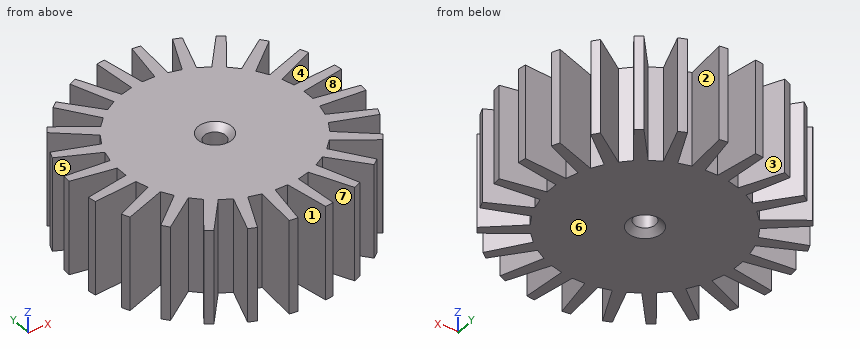
from build123d import *

# Parameters (mm, degrees)
SKETCH_R           = 22
PAD_DEPTH          = 15
SKETCH001_R        = 1.7
POCKET_DEPTH       = 15.001
POCKET001_DEPTH    = 143.016624
POLARPATTERN_COUNT = 24
CHAMFER_SIZE       = 1


with BuildPart() as part:
    # Sketch → Pad (new body)
    with BuildSketch(Plane.XY):
        Circle(SKETCH_R)
    extrude(amount=PAD_DEPTH)

    # Sketch001 (on Face3 of Pad) → Pocket (cut, through all)
    with BuildSketch(Plane.XY.offset(15)):
        Circle(SKETCH001_R)
    extrude(amount=-POCKET_DEPTH, mode=Mode.SUBTRACT)

    # Sketch002 (on Face3 of Pocket) → Pocket001 (cut, through all)
    with BuildSketch(Plane.XY.offset(15)):
        Polygon((-1, 15), (1, 15), (4.820269, 36.665769), (-4.820254, 36.665772), align=None)
    pocket001 = extrude(amount=-POCKET001_DEPTH, mode=Mode.SUBTRACT)

    # PolarPattern: Pocket001 ×24 about axis
    polarpattern_axis = Axis((0, 0, 0), (0, 0, 1))
    for i in range(1, POLARPATTERN_COUNT):
        add(pocket001.rotate(polarpattern_axis, i * 360 / POLARPATTERN_COUNT), mode=Mode.SUBTRACT)

    # Chamfer
    chamfer_edges = [part.edges().sort_by_distance(p)[0] for p in [
        (-1.7, 0, 15),
        (-1.7, 0, 0),
    ]]
    chamfer(chamfer_edges, length=CHAMFER_SIZE)


solid = part.part
Input: part model. Units: mm. Frame: model coordinates. Face numbers are marked on the shaded views. A direction names the side the tool comes from. Round coordinates to 2 decimals unless told otherwise and drop trailing zeros. Order: outer loops, then holes, each group sorted by start corner. A loop starts at its lowest first (then second) coordinate and runs counter-clockwise, first axis right, second up.
1. Material intervals for line 1 (Y direction, x = 0, z = 10); line 2 (X direction, y = 18.5, z = 2.5); line 3 (Y direction, x = 13.5, z = 11.5), sorted ascending.
The answers:
line 1: y = -15 to -1.7, 1.7 to 15
line 2: x = -8.46 to -6.84, -3.24 to -1.62, 1.62 to 3.24, 6.84 to 8.46
line 3: y = -17.37 to -16.46, -11.43 to -9.21, -6.64 to 6.64, 9.21 to 11.43, 16.46 to 17.37
2. Set-up query: the marked faces 1, 2, 3 and 4. Return all of +Z, -Z, +X, -X, +Y, -Y with unobstructed straight access to the full face (end or side cutting, diameter ignored); none if empty.
The answers:
face 1: +Z, -Z, -Y
face 2: +Z, -Z
face 3: +Z, -Z, +Y
face 4: +Z, -Z, +X
3. Mould query, pull axis X, two halves, no side actions, for the marked faces 5, 6, 7 and 8. Classes: released by +X, released by -X, zero draft, split by the parting line, or undercut.
The answers:
face 5: released by -X
face 6: zero draft
face 7: undercut
face 8: released by +X
4. Cut plane A-A, the plane y = 0. Output: boundary loops of the cut face in (x, z), then the cut area to 3 significant figures.
The answers:
outline: (-15, 0) - (-2.7, 0) - (-1.7, 1) - (-1.7, 14) - (-2.7, 15) - (-15, 15) - close; (1.7, 1) - (2.7, 0) - (15, 0) - (15, 15) - (2.7, 15) - (1.7, 14) - close
area: 397 mm2
5. Cut plane C-C, the plane x = 19. Output: boundary loops of the cut face in (y, z).
The answers:
outline: (-8.64, 0) - (-7.07, 0) - (-7.07, 15) - (-8.64, 15) - close; (-3.29, 0) - (-1.71, 0) - (-1.71, 15) - (-3.29, 15) - close; (1.71, 0) - (3.29, 0) - (3.29, 15) - (1.71, 15) - close; (7.07, 0) - (8.64, 0) - (8.64, 15) - (7.07, 15) - close
6. Pin query (flat end, axial travel): P1, Ø1, axis at y = -17, z = 2.5, coming from the +X side; P2, Ø4, axis at x = -15.5, z = 3, coming from the +Y side; P3, Ø1, axis at x = -11.5, z = 11, coming from the -Y side. Return the tip coordinate at first contact, or that it passes through.
The answers:
P1: stops at x = 13.91
P2: stops at y = 17.37
P3: stops at y = -16.82
